```python
from build123d import *

# Parameters (mm, degrees)
F1_R     = 10
F2_DEPTH = 6
F0_R     = 5
F0_R_2   = 4.5
F0_R_3   = 1.75
F3_DEPTH = 6
F4_DEPTH = 6
F7_DEPTH = 12


# Not quite as in the source:
# - the program builds the solid bodies; features that only make, move or delete a surface that nothing else refers to are left out


with BuildPart() as f2:
    # F1 (on Top) → F2 (new body)
    with BuildSketch(Plane.XY):
        Circle(F1_R)
    extrude(amount=F2_DEPTH)

    # F0 (on Top) → F3 (cut, symmetric)
    with BuildSketch(Plane.XY):
        Circle(F0_R)
        Circle(F0_R_2, mode=Mode.SUBTRACT)
        with Locations((0, 7.5)):
            Circle(F0_R_3)
        with Locations((-7.5, 0)):
            Circle(F0_R_3)
        with Locations((0, -7.5)):
            Circle(F0_R_3)
        with Locations((7.5, 0)):
            Circle(F0_R_3)
    extrude(amount=F3_DEPTH, both=True, mode=Mode.SUBTRACT)

    # F4 (cut): a face of the model
    f4_faces = [f2.faces().sort_by_distance(p)[0] for p in [
        (0, 0, 6),
    ]]
    extrude(f4_faces, amount=-F4_DEPTH, mode=Mode.SUBTRACT)

    # F0 (on Top) → F7 (join)
    with BuildSketch(Plane.XY):
        Circle(F0_R)
        Circle(F0_R_2, mode=Mode.SUBTRACT)
    extrude(amount=F7_DEPTH)


solid = f2.part
```
Part model, mm, in its own coordinate system. A direction names the side the tool comes from. Round coordinates to 2 decimals unless told otherwise and drop trailing zeros. Write each loop counter-clockwise with the first axis right and the second up, starting at its lowest first coordinate (ties: lowest second). Pieces come first, ordered by that corner, then holes. Notation, with made-up numbers: M 10,0 L 33,0 A28 cw 33,36 Z; hole C 81,-4.5 d10. An arc over 180 degrees is marked long. Answer as CSV lines item,"result". Start each with the question number.
1) Which spindle directions (+Z, -Z, +X, -X, +Y, -Y) get a long thin tool onto all of the face, cutting with end or side? Do faces 1 (the face through (-5.831, 0.526, 2.958)), 2 (the face through (-5, -2, 6)). Say none if no direction does.
2) Band-saw the part on C-C (z = 4.5). List the corners of the cut face in (x, y).
3) Drop flat-ended pins along their axis: pin 1 (2 mm diameter, centred on x = 0, y = 7.5, fed in from +Z); pin 2 (4 mm diameter, centred on x = -2, z = 10, fed in from -Y); pin 3 (1 mm diameter, centred on y = -5.5, z = 3, fed in from +X); pin 4 (1 mm diameter, centred on x = -4.5, z = 1.5, fed in from -Y). Give the stop position or say it passes through.
4) Drill centre lines: L1, parallel to Y at x = 0, z = 2.6; L2, parallel to X at y = -1.5, z = 2.25; L3, parallel to Z at x = 8, y = -2.25. Where is each one in solid material? Low to high.
5) Band-saw the part on A-A (x = 0). List the corners of the cut face in (y, z), then the cut area to 3 significant figures.
6) Band-saw the part on D-D (x = 8.75). List the corners of the cut face in (y, z), then the cut area to 3 significant figures.
7) Mould opens along Y. For faces 3 (the face through (4.3, -2.1, 0)), 4 (the face through (-1.08, -4.88, 8.96)), 5 (the face through (-0.38, 5.79, 2.96)) say: +Y half, -Y half, draft (parallel to the pull), parting line (faces both ways), or undercut.
Worked out:
1,face 1,"+Z, -Z"
1,face 2,"+Z"
2,outline,"C 0,0 d20; hole C -7.5,0 d3.5; hole C 0,0 d9; hole C 0,-7.5 d3.5; hole C 0,7.5 d3.5; hole C 7.5,0 d3.5"
3,pin 1,"through"
3,pin 2,"y = -5"
3,pin 3,"x = 8.66"
3,pin 4,"y = -9.17"
4,L1,"-10 to -9.25, -5.75 to -4.5, 4.5 to 5.75, 9.25 to 10"
4,L2,"-9.89 to -8.4, -6.6 to -4.24, 4.24 to 6.6, 8.4 to 9.89"
4,L3,"0 to 6"
5,outline,"M -10,0 L -9.25,0 L -9.25,6 L -10,6 Z; M -5.75,0 L -4.5,0 L -4.5,12 L -5,12 L -5,6 L -5.75,6 Z; M 4.5,0 L 5.75,0 L 5.75,6 L 5,6 L 5,12 L 4.5,12 Z; M 9.25,0 L 10,0 L 10,6 L 9.25,6 Z"
5,area,"30.0 mm²"
6,outline,"M -4.84,0 L -1.22,0 L -1.22,6 L -4.84,6 Z; M 1.22,0 L 4.84,0 L 4.84,6 L 1.22,6 Z"
6,area,"43.4 mm²"
7,face 3,"draft"
7,face 4,"parting line"
7,face 5,"undercut"
